```python
from build123d import *

# Parameters (mm, degrees)
SKETCH2_R           = 1
SKETCH2_R_2         = 5
SKETCH2_W           = 5.4
SKETCH2_H           = 5.4
BOSS_EXTRUDE1_DEPTH = 5


with BuildPart() as part:
    # Sketch2 → Boss-Extrude1 (new body)
    with BuildSketch(Plane.XY):
        with BuildLine():
            Line((-5.74908406, 12.042291654), (44.25091594, 12.042291654))
            Line((44.25091594, 12.042291654), (44.25091594, -7.457708346))
            Line((44.25091594, -7.457708346), (-5.74908406, -7.457708346))
            ThreePointArc((-5.74908406, -7.457708346), (-15.49908406, 2.292291654), (-5.74908406, 12.042291654))
        make_face()
        with Locations((-5.811538636, 9.292291654)):
            Circle(SKETCH2_R, mode=Mode.SUBTRACT)
        with Locations((-10.742794828, 7.197681829)):
            Circle(SKETCH2_R, mode=Mode.SUBTRACT)
        with Locations((-12.74908406, 2.229837079)):
            Circle(SKETCH2_R, mode=Mode.SUBTRACT)
        with Locations((-0.843693885, 7.286002421)):
            Circle(SKETCH2_R, mode=Mode.SUBTRACT)
        with Locations((1.25091594, 2.354746229)):
            Circle(SKETCH2_R, mode=Mode.SUBTRACT)
        with Locations((-0.755373293, -2.613098521)):
            Circle(SKETCH2_R, mode=Mode.SUBTRACT)
        with Locations((-5.686629485, -4.707708346)):
            Circle(SKETCH2_R, mode=Mode.SUBTRACT)
        with Locations((-10.654474236, -2.701419114)):
            Circle(SKETCH2_R, mode=Mode.SUBTRACT)
        with Locations((-5.74908406, 2.292291654)):
            Circle(SKETCH2_R_2, mode=Mode.SUBTRACT)
        with Locations((37.55091594, 7.092291654)):
            Rectangle(SKETCH2_W, SKETCH2_H, mode=Mode.SUBTRACT)
        with Locations((37.55091594, -2.507708346)):
            Rectangle(SKETCH2_W, SKETCH2_H, mode=Mode.SUBTRACT)
    extrude(amount=BOSS_EXTRUDE1_DEPTH)


solid = part.part
```
The listing builds one solid part. Answer for the finished solid, in the listing's coordinates (mm). A direction names the side the tool comes from. Give positions to 0.01 mm unless a question says otherwise; leave off trailing zeros. Order: outer loops, then holes, each group sorted by start corner. A loop starts at its lowest first (then second) coordinate and runs counter-clockwise, first axis right, second up. Notation, with made-up numbers: (-40, 53.5) -> (12, 53.5) arc R22 ccw to (12, 84.5) -> close; hole circle Ø5 at (29, 25.5). An arc over 180 degrees is marked (long way). Answer as CSV lines item,"result". Start each with the question number.
Q1. Determine the mould class of faces 3 (the flat face through (15, 2, 0)), 4 (the cylindrical face through (-4.73, -4.41, 2.46)), 5 (the flat face through (20, -7.458, 2)), 6 (the cylindrical face through (-0.886, -1.622, 2.465)) for opening direction Y: pulls with the +Y half, pulls with the -Y half, needs draft (parallel to the pull), parting line crosses it, or undercut.
Q2. A cutting plane is placed at C-C (x = -8.5). Determine the outline of the cut face in (y, z).
Q3. A cutting plane is placed at B-B (y = -0.75). Determine the outline of the cut face in (x, z).
Q4. Which of the six approach directions +Z, -Z, +X, -X, +Y, -Y give full straight-line access (tool end or side, diameter ignored) to faces 1 (the flat face through (40.251, -3, 2)), 2 (the cylindrical face through (-15.497, 2.078, 2.465))?
Q5. A cutting plane is placed at A-A (x = 38). Determine the outline of the cut face in (y, z).
Q6. Find the intervals of material crossed by L1, parallel to X at y = 8.5, z = 0.75; L2, parallel to Y at x = 37.5, z = 0.6; L3, parallel to Y at x = -6, z = 1.65, in increasing order.
Q7. Given pin 1 (1.5 mm diameter, centred on y = -1.5, z = 2.5, fed in from -X); pin 2 (2.5 mm diameter, centred on y = 6, z = 3.5, fed in from -X), each flat-ended and moving along its own axis, determine where each tip first touches the part or whether it passes through.
Q8. A cutting plane is placed at D-D (z = 4.15). Count the separate pieces of the cut face and the enclosed holes in it, then the cut area to 3 significant figures.
Results found:
1,face 3,"needs draft"
1,face 4,"undercut"
1,face 5,"pulls with the -Y half"
1,face 6,"undercut"
2,outline,"(-7.06, 0) -> (-1.88, 0) -> (-1.88, 5) -> (-7.06, 5) -> close; (6.47, 0) -> (11.65, 0) -> (11.65, 5) -> (6.47, 5) -> close"
3,outline,"(-15.01, 0) -> (-9.72, 0) -> (-9.72, 5) -> (-15.01, 5) -> close; (-1.78, 0) -> (34.85, 0) -> (34.85, 5) -> (-1.78, 5) -> close; (40.25, 0) -> (44.25, 0) -> (44.25, 5) -> (40.25, 5) -> close"
4,face 1,"+Z, -Z"
4,face 2,"+Z, -Z, -X"
5,outline,"(-7.46, 0) -> (-5.21, 0) -> (-5.21, 5) -> (-7.46, 5) -> close; (0.19, 0) -> (4.39, 0) -> (4.39, 5) -> (0.19, 5) -> close; (9.79, 0) -> (12.04, 0) -> (12.04, 5) -> (9.79, 5) -> close"
6,L1,"-13.27 to -6.42, -5.2 to 34.85, 40.25 to 44.25"
6,L2,"-7.46 to -5.21, 0.19 to 4.39, 9.79 to 12.04"
6,L3,"-7.45 to -5.66, -3.76 to -2.7, 7.29 to 8.31, 10.27 to 12.04"
7,pin 1,"x = -15.01"
7,pin 2,"x = -15.18"
8,separate pieces,"1"
8,enclosed holes,"11"
8,area,"962 mm2"
